from build123d import *

# Parameters (mm, degrees)
SKETCH1_R           = 65
SKETCH1_R_2         = 16.15
SKETCH1_R_3         = 2.4
SKETCH1_R_4         = 4
SKETCH1_R_5         = 1.475
SKETCH1_W           = 50
SKETCH1_H           = 5
BOSS_EXTRUDE1_DEPTH = 5


with BuildPart() as part:
    # Sketch1 → Boss-Extrude1 (new body)
    with BuildSketch(Plane.XY):
        Circle(SKETCH1_R)
        Circle(SKETCH1_R_2, mode=Mode.SUBTRACT)
        with Locations((0, 52)):
            Circle(SKETCH1_R_3, mode=Mode.SUBTRACT)
        with Locations((-30, 0)):
            Circle(SKETCH1_R_3, mode=Mode.SUBTRACT)
        with Locations((0, -52)):
            Circle(SKETCH1_R_3, mode=Mode.SUBTRACT)
        with Locations((30, 0)):
            Circle(SKETCH1_R_3, mode=Mode.SUBTRACT)
        with Locations((-41.365746699, 41.365746699)):
            Circle(SKETCH1_R_4, mode=Mode.SUBTRACT)
        with Locations((-29.25, 50.662486121)):
            Circle(SKETCH1_R_4, mode=Mode.SUBTRACT)
        with Locations((-50.662486121, 29.25)):
            Circle(SKETCH1_R_4, mode=Mode.SUBTRACT)
        with Locations((50.662486121, 29.25)):
            Circle(SKETCH1_R_4, mode=Mode.SUBTRACT)
        with Locations((41.365746699, 41.365746699)):
            Circle(SKETCH1_R_4, mode=Mode.SUBTRACT)
        with Locations((29.25, 50.662486121)):
            Circle(SKETCH1_R_4, mode=Mode.SUBTRACT)
        with Locations((50.662486121, -29.25)):
            Circle(SKETCH1_R_4, mode=Mode.SUBTRACT)
        with Locations((41.365746699, -41.365746699)):
            Circle(SKETCH1_R_4, mode=Mode.SUBTRACT)
        with Locations((29.25, -50.662486121)):
            Circle(SKETCH1_R_4, mode=Mode.SUBTRACT)
        with Locations((-29.25, -50.662486121)):
            Circle(SKETCH1_R_4, mode=Mode.SUBTRACT)
        with Locations((-41.365746699, -41.365746699)):
            Circle(SKETCH1_R_4, mode=Mode.SUBTRACT)
        with Locations((-50.662486121, -29.25)):
            Circle(SKETCH1_R_4, mode=Mode.SUBTRACT)
        with Locations((-40, 10)):
            Circle(SKETCH1_R_5, mode=Mode.SUBTRACT)
        with Locations((-50, 10)):
            Circle(SKETCH1_R_5, mode=Mode.SUBTRACT)
        with Locations((-40, -10)):
            Circle(SKETCH1_R_5, mode=Mode.SUBTRACT)
        with Locations((-50, -10)):
            Circle(SKETCH1_R_5, mode=Mode.SUBTRACT)
        with Locations((50, -10)):
            Circle(SKETCH1_R_5, mode=Mode.SUBTRACT)
        with Locations((40, -10)):
            Circle(SKETCH1_R_5, mode=Mode.SUBTRACT)
        with Locations((40, 10)):
            Circle(SKETCH1_R_5, mode=Mode.SUBTRACT)
        with Locations((50, 10)):
            Circle(SKETCH1_R_5, mode=Mode.SUBTRACT)
        with Locations((0, -22.5)):
            Rectangle(SKETCH1_W, SKETCH1_H, mode=Mode.SUBTRACT)
        with Locations((0, 22.5)):
            Rectangle(SKETCH1_W, SKETCH1_H, mode=Mode.SUBTRACT)
    extrude(amount=BOSS_EXTRUDE1_DEPTH)


solid = part.part
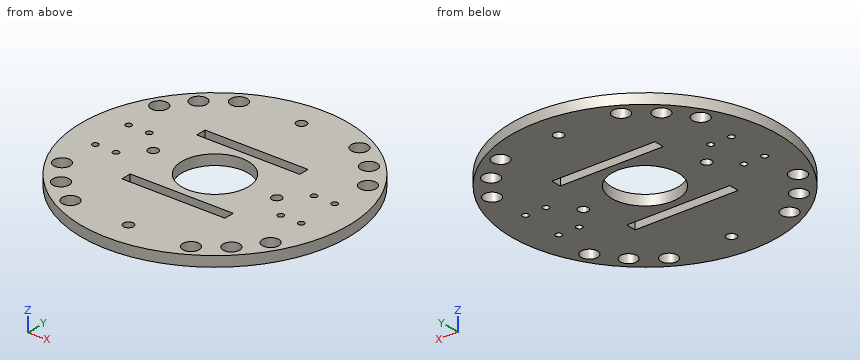
Can you work these out from the model? Positions are in its coordinate system, mm. Give positions to 0.01 mm unless a question says otherwise; leave off trailing zeros. Loops run counter-clockwise (first coordinate to the right, second up) from the corner with the lowest first, then second, coordinate; pieces in that order, holes last. Notation, with made-up numbers: M -25,-5.75 L 31,-5.75 A17 cw 31,24.25 Z; hole C 10,18.5 d8. An arc over 180 degrees is marked long. One line per item, written item: value. Start each with the question number.
1) If we section it at D-D, the plane y = -5: Write out the boundary of the cut face in (x, z).
2) I'm going to push flat-ended pins straight in: pin 1 (2 mm diameter, centred on x = -31.5, z = 1.5, fed in from -Y); pin 2 (1.5 mm diameter, centred on y = -43.5, z = 3, fed in from -X). Where does each tip first touch, or does it pass through?
3) If I drill on line 1 (Y direction, x = 0, z = 2.4); line 2 (Y direction, x = -48, z = 4.6); line 3 (X direction, y = -10.5, z = 4.4), over which ranges is the centre line in solid material (lowest first)? Write a range as [from, to].
4) If we section it at C-C, the plane x = 29.25: Write out the boundary of the cut face in (y, z).
5) If we section it at A-A, the plane x = 0: Write out the boundary of the cut face in (y, z).
6) If we section it at B-B, the plane y = 43.5: Write out the boundary of the cut face in (x, z).
Completed:
1. outline: M -64.81,0 L -15.36,0 L -15.36,5 L -64.81,5 Z; M 15.36,0 L 64.81,0 L 64.81,5 L 15.36,5 Z
2. pin 1: stops at y = -57.4
2. pin 2: stops at x = -48.96
3. line 1: y = [-65, -54.4], [-49.6, -25], [-20, -16.15], [16.15, 20], [25, 49.6], [54.4, 65]
3. line 2: y = [-43.83, -32.24], [-26.26, 26.26], [32.24, 43.83]
3. line 3: x = [-64.15, -51.39], [-48.61, -41.39], [-38.61, -12.27], [12.27, 38.61], [41.39, 48.61], [51.39, 64.15]
4. outline: M -58.05,0 L -54.66,0 L -54.66,5 L -58.05,5 Z; M -46.66,0 L -2.28,0 L -2.28,5 L -46.66,5 Z; M 2.28,0 L 46.66,0 L 46.66,5 L 2.28,5 Z; M 54.66,0 L 58.05,0 L 58.05,5 L 54.66,5 Z
5. outline: M -65,0 L -54.4,0 L -54.4,5 L -65,5 Z; M -49.6,0 L -25,0 L -25,5 L -49.6,5 Z; M -20,0 L -16.15,0 L -16.15,5 L -20,5 Z; M 16.15,0 L 20,0 L 20,5 L 16.15,5 Z; M 25,0 L 49.6,0 L 49.6,5 L 25,5 Z; M 54.4,0 L 65,0 L 65,5 L 54.4,5 Z
6. outline: M -48.3,0 L -44.75,0 L -44.75,5 L -48.3,5 Z; M -37.98,0 L 37.98,0 L 37.98,5 L -37.98,5 Z; M 44.75,0 L 48.3,0 L 48.3,5 L 44.75,5 Z
